Input: part model. Units: mm. Frame: model coordinates. A direction names the side the tool comes from. Give positions to 0.01 mm unless a question says otherwise; leave off trailing zeros. Loops run counter-clockwise (first coordinate to the right, second up) from the corner with the lowest first, then second, coordinate; pieces in that order, holes last. Notation, with made-up numbers: (-35, 32.5) - (10, 32.5) arc R18 cw to (10, 63.5) - close; hole circle Ø11 at (-5.75, 87). An arc over 180 degrees is marked (long way). Answer as a JSON object with one key per item and string values. Group by question number.
(1) Mould query, pull axis Z, two halves, no side actions, for faces 3 (the flat face through (1.9, 44, -8)), 4 (the cylindrical face through (1.802, 37.08, 5.723)), 5 (the flat face through (0, 43.1, 0)). Classes: +Z half, -Z half, draft (parallel to the pull), parting line (faces both ways), or undercut.
(2) Material intervals for L1, parallel to Y at x = -0.75, z = -3.75; L2, parallel to X at y = 42, z = -7; L3, parallel to Y at x = 0.25, z = -1.5, sorted ascending.
(3) Access query for faces 1 (the cylindrical face through (0.9, 17.5, 2.86)), 2 (the flat face through (-0.027, 48.596, -9.076)). Directions: +Z, -Z, +X, -X, +Y, -Y. A direction counts if a zero-diameter tool reaches every point of the face in a straight line with its end or side. Return the directions, or none.
(4) Pin query (flat end, axial travel): P1, Ø6, axis at y = 20, z = 1, coming from the +X side; P2, Ø7.5, axis at y = 43, z = -6, coming from the -X side; P3, Ø2, axis at y = 44, z = 6.5, coming from the +X side. Return the tip coordinate at first contact, or that it passes through.
(5) Section query A-A (y = 20). Return loops of the section in (x, z).
```python
from build123d import *

# Parameters (mm, degrees)
SKETCH_1_R           = 3
EXTRUDE_1_DEPTH      = 35.5
SKETCH_2_R           = 6
EXTRUDE_2_DEPTH      = 3
FILLET_1_R           = 0.2
EXTRUDE_3_DEPTH      = 1.9
EXTRUDE_3_DEPTH_BACK = 1.9


with BuildPart() as part:
    # Sketch 1 → Extrude 1 (new body)
    with BuildSketch(Plane(origin=(0, 0, 0), x_dir=(1, 0, 0), z_dir=(0, 1, 0))):
        with Locations(Location((0, 0, 0), (0, 0, 270))):
            Circle(SKETCH_1_R)
    extrude(amount=EXTRUDE_1_DEPTH)

    # Sketch 2 → Extrude 2 (add)
    with BuildSketch(Plane(origin=(0, 35.5, 0), x_dir=(1, 0, 0), z_dir=(0, 1, 0))):
        with Locations(Location((0, 0, 0), (0, 0, 270))):
            Circle(SKETCH_2_R)
    extrude(amount=EXTRUDE_2_DEPTH)

    # Sketch 3 → Revolve 1 (revolve)
    with BuildSketch(Plane(origin=(0, 0, 0), x_dir=(0, 0, -1), z_dir=(1, 0, 0))):
        Polygon((0, 43.1), (4.4, 43.1), (6.5, 40), (6, 38.5), (0, 38.5), align=None)
    revolve(axis=Axis((0, 38.5, 0), (0, 1, 0)))

    # Fillet 1
    fillet_1_edges = [part.edges().sort_by_distance(p)[0] for p in [
        (0, 35.5, -6),
        (0, 43.1, 4.4),
        (0, 40, 6.5),
    ]]
    fillet(fillet_1_edges, radius=FILLET_1_R)

    # Sketch 4 → Extrude 3 (add, two sides: drawn at the far end of the back side and taken through both)
    with BuildSketch(Plane(origin=(0, 0, 0), x_dir=(0, 0, -1), z_dir=(1, 0, 0)).offset(-EXTRUDE_3_DEPTH_BACK)):
        with BuildLine():
            Line((7.129672899, 49.216052305), (11.078140475, 47.958388396))
            add(Edge.make_bspline(
                [(11.078140475, 47.958388396), (10.847677477, 46.568474241), (10.449817168, 45.302296098), (9.907358884, 43.260826265), (9.311295548, 41.6663192), (8.235465928, 40.02121413), (7.619812039, 39.286169598), (6.4951686, 38.593529849), (6, 38.5)],
                knots=[0, 0, 0, 0, 0.303156728, 0.355873298, 0.527165706, 0.682347727, 0.853387488, 1, 1, 1, 1], degree=3))
            Line((6, 38.5), (4.293914255, 43.1))
            add(Edge.make_bspline(
                [(4.293914255, 43.1), (4.703822543, 43.319985303), (4.99322637, 42.768371987), (6.293739819, 46.611799248), (7.129672899, 49.216052305)],
                knots=[0, 0, 0, 0, 0.337975892, 1, 1, 1, 1], degree=3))
        make_face()
        with BuildLine():
            Line((-4.293914255, 43.1), (-6, 38.5))
            add(Edge.make_bspline(
                [(-11.078140475, 47.958388396), (-10.847677477, 46.568474241), (-10.449817168, 45.302296098), (-9.907358884, 43.260826265), (-9.311295548, 41.6663192), (-8.235465928, 40.02121413), (-7.619812039, 39.286169598), (-6.4951686, 38.593529849), (-6, 38.5)],
                knots=[0, 0, 0, 0, 0.303156728, 0.355873298, 0.527165706, 0.682347727, 0.853387488, 1, 1, 1, 1], degree=3))
            Line((-11.078140475, 47.958388396), (-7.129672899, 49.216052305))
            add(Edge.make_bspline(
                [(-4.293914255, 43.1), (-4.703822543, 43.319985303), (-4.99322637, 42.768371987), (-6.293739819, 46.611799248), (-7.129672899, 49.216052305)],
                knots=[0, 0, 0, 0, 0.337975892, 1, 1, 1, 1], degree=3))
        make_face()
    extrude(amount=EXTRUDE_3_DEPTH + EXTRUDE_3_DEPTH_BACK)


solid = part.part
```
Recorded:
{
 "1": {"face 3": "draft", "face 4": "parting line", "face 5": "undercut"},
 "2": {"L1": "y = 35.5 to 43.1", "L2": "x = -1.9 to 1.9", "L3": "y = 0 to 43.1"},
 "3": {"face 1": "-Y", "face 2": "-Z, +X, -X, +Y"},
 "4": {"P1": "stops at x = 3", "P2": "stops at x = -5.32", "P3": "stops at x = 1.9"},
 "5": {"outline": "circle Ø6 at (0, 0)"}
}
